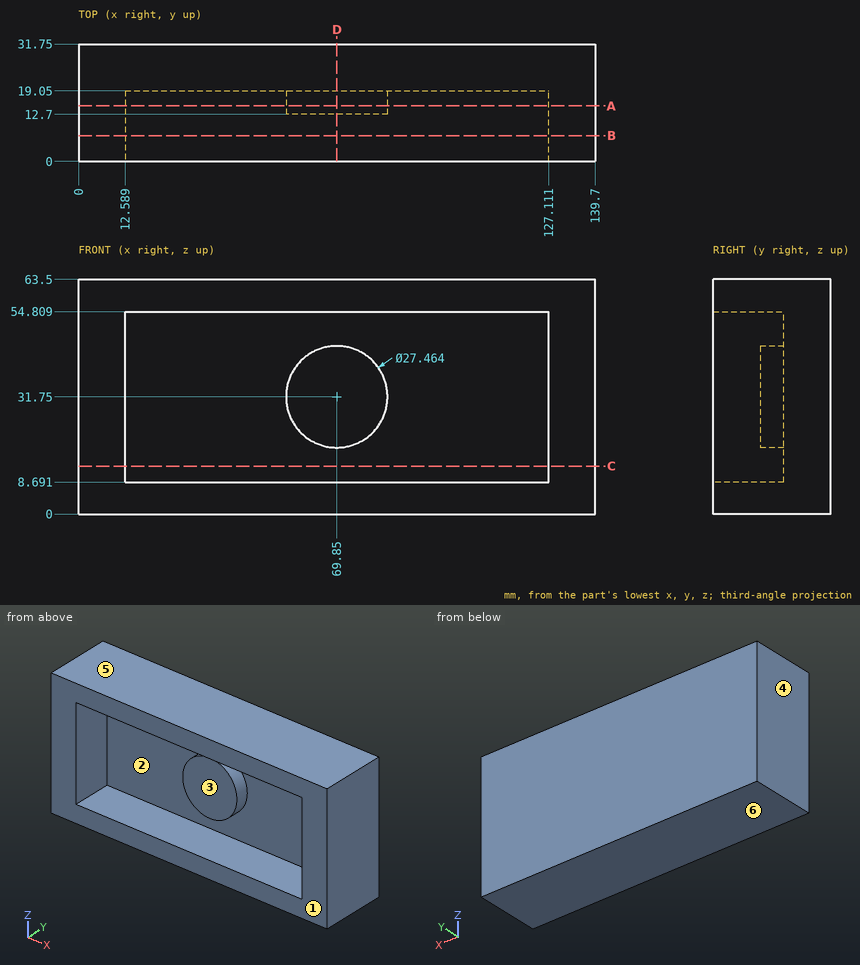
Verification items for this drawing (mm, ordinates from the low corner). A direction names the side the tool comes from. Give positions to 0.01 mm unless a question says otherwise; leave off trailing zeros. Write each loop counter-clockwise with the first axis right and the second up, starting at its lowest first coordinate (ties: lowest second). Pieces come first, ordered by that corner, then holes. Notation, with made-up numbers: (61, 15.5) - (107, 15.5) arc R6 ccw to (107, 20.5) - close; hole circle Ø6 at (44, 76). An arc over 180 degrees is marked (long way). Answer as a JSON object with one key per item and string values. Group by question number.
1) Sectioned sample at D-D (x = 69.85). Record the cut outline in (y, z).
2) Sectioned sample at C-C (z = 13). Record the cut outline in (x, y), then the cut area to 3 significant figures.
3) Sectioned sample at A-A (y = 15). Record the cut outline in (x, z).
4) Sectioned sample at B-B (y = 7). Record the cut outline in (x, z).
5) Depth check by flat-ended pin: P1, Ø12, axis at x = 26, z = 34.5, coming from the -Y side; P2, Ø14, axis at x = 87, z = 24, coming from the -Y side. Enter the tip coordinate at first touch or a pass-through.
6) Access from +Z, -Z, +X, -X, +Y, -Y to the whole of each face (thin tool, end or side, straight path). Record for the marked faces 1 and 2.
7) Release check for a two-part mould opening along Z. For the marked faces 3, 4, 5 and 6 record: pulls with the +Z half, pulls with the -Z half, needs draft (parallel to the pull), parting line crosses it, or undercut.
8) Thickness scan on probe 1 along Z at (x, y) = (91.5, 7.5); probe 2 along X at (y, z) = (18.5, 49); probe 3 along Z at (x, y) = (61.5, 18). Record the ranges inside material, lowest first. Write a range as from..to.
Geometry results:
{
 "1": {"outline": "(0, 0) - (31.75, 0) - (31.75, 63.5) - (0, 63.5) - (0, 54.81) - (19.05, 54.81) - (19.05, 45.48) - (12.7, 45.48) - (12.7, 18.02) - (19.05, 18.02) - (19.05, 8.69) - (0, 8.69) - close"},
 "2": {"outline": "(0, 0) - (12.59, 0) - (12.59, 19.05) - (127.11, 19.05) - (127.11, 0) - (139.7, 0) - (139.7, 31.75) - (0, 31.75) - close", "area": "2,250 mm^2"},
 "3": {"outline": "(0, 0) - (139.7, 0) - (139.7, 63.5) - (0, 63.5) - close; circle Ø27.46 at (69.85, 31.75); hole (12.59, 8.69) - (127.11, 8.69) - (127.11, 54.81) - (12.59, 54.81) - close"},
 "4": {"outline": "(0, 0) - (139.7, 0) - (139.7, 63.5) - (0, 63.5) - close; hole (12.59, 8.69) - (127.11, 8.69) - (127.11, 54.81) - (12.59, 54.81) - close"},
 "5": {"P1": "stops at y = 19.05", "P2": "stops at y = 12.7"},
 "6": {"face 1": "+Z, -Z, +X, -X, -Y", "face 2": "-Y"},
 "7": {"face 3": "undercut", "face 4": "needs draft", "face 5": "pulls with the +Z half", "face 6": "pulls with the -Z half"},
 "8": {"probe 1": "z = 0..8.69, 54.81..63.5", "probe 2": "x = 0..12.59, 127.11..139.7", "probe 3": "z = 0..8.69, 20.85..42.65, 54.81..63.5"}
}
